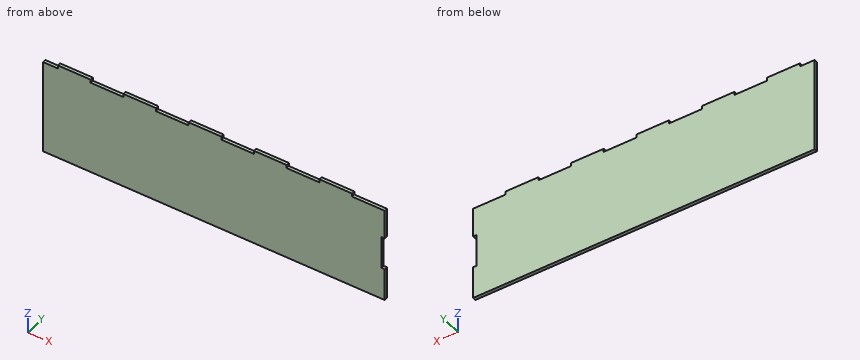
from build123d import *

# Parameters (mm, degrees)
SKETCH1_W              = 630
SKETCH1_H              = 90
BOSS_EXTRUDE1_DEPTH    = 3
SKETCH3_W              = 30
SKETCH3_H              = 3
CUT_EXTRUDE1_DEPTH     = 3
LPATTERN1_COUNT        = 10
LPATTERN1_PITCH        = 60
LPATTERN1_COL_COUNT    = 2
LPATTERN1_COL_PITCH    = 60
CUT_EXTRUDE5_START     = -3
CUT_EXTRUDE5_OUTLINE_W = 3
CUT_EXTRUDE5_OUTLINE_H = 30
CUT_EXTRUDE5_DEPTH     = 3
SKETCH7_W              = 3
SKETCH7_H              = 30
CUT_EXTRUDE3_DEPTH     = 3
SKETCH13_W             = 3
SKETCH13_H             = 27
CUT_EXTRUDE4_DEPTH     = 10


# Read off the part's stored shape, not the designer's step: Cut-Extrude5
with BuildPart() as part:
    # Sketch1 → Boss-Extrude1 (new body)
    with BuildSketch(Plane(origin=(0, 0, 0), x_dir=(1, 0, 0), z_dir=(0, 1, 0))):
        Rectangle(SKETCH1_W, SKETCH1_H)
    extrude(amount=BOSS_EXTRUDE1_DEPTH)

    # Sketch3 → Cut-Extrude1 (cut)
    with BuildSketch(Plane(origin=(0, 3, 0), x_dir=(1, 0, 0), z_dir=(0, 1, 0))):
        with Locations((-240, -43.5)):
            Rectangle(SKETCH3_W, SKETCH3_H)
    cut_extrude1 = extrude(amount=-CUT_EXTRUDE1_DEPTH, mode=Mode.SUBTRACT)

    # LPattern1: Cut-Extrude1 ×10
    with Locations(*[(i * LPATTERN1_PITCH, 0, 0) for i in range(1, LPATTERN1_COUNT)]):
        add(cut_extrude1, mode=Mode.SUBTRACT)

    # LPattern1 col: Cut-Extrude1 ×2
    with Locations(*[(-i * LPATTERN1_COL_PITCH, 0, 0) for i in range(1, LPATTERN1_COL_COUNT)]):
        add(cut_extrude1, mode=Mode.SUBTRACT)

    # Cut-Extrude5 outline → Cut-Extrude5 (cut)
    with BuildSketch(Plane(origin=(0, 3, 0), x_dir=(1, 0, 0), z_dir=(0, 1, 0)).offset(CUT_EXTRUDE5_START)):
        with Locations((313.5, 1e-09)):
            Rectangle(CUT_EXTRUDE5_OUTLINE_W, CUT_EXTRUDE5_OUTLINE_H)
    extrude(amount=CUT_EXTRUDE5_DEPTH, mode=Mode.SUBTRACT)

    # Sketch7 → Cut-Extrude3 (cut)
    with BuildSketch(Plane(origin=(0, 3, 0), x_dir=(1, 0, 0), z_dir=(0, 1, 0))):
        with Locations((-313.5, 30)):
            Rectangle(SKETCH7_W, SKETCH7_H)
    extrude(amount=-CUT_EXTRUDE3_DEPTH, mode=Mode.SUBTRACT)

    # Sketch13 → Cut-Extrude4 (cut)
    with BuildSketch(Plane(origin=(0, 3, 0), x_dir=(1, 0, 0), z_dir=(0, 1, 0))):
        with Locations((-313.5, -28.5)):
            Rectangle(SKETCH13_W, SKETCH13_H)
    extrude(amount=-CUT_EXTRUDE4_DEPTH, mode=Mode.SUBTRACT)

    # SurfaceCut1
    split(bisect_by=Plane.ZY.offset(-1.295), keep=Keep.BOTTOM)


solid = part.part
Here's how the part is built. I have some questions about the finished solid (model axes, mm). Give positions to 0.01 mm unless a question says otherwise; leave off trailing zeros. Loops run counter-clockwise (first coordinate to the right, second up) from the corner with the lowest first, then second, coordinate; pieces in that order, holes last. Notation, with made-up numbers: (86, 41.25) -> (95, 41.25) arc R23 ccw to (95, 59.25) -> close; hole circle Ø5 at (-21, 71). An arc over 180 degrees is marked (long way). One line per item, written item: value.
Q1. I'm going to push flat-ended pins straight in: pin 1 Ø1.5 at (y, z) = (1, 43.5) entering from +X; pin 2 Ø1.5 at (y, z) = (2, 44) entering from -X; pin 3 Ø1.5 at (x, y) = (300, 1.5) entering from +Z. Where does each tip first touch, or does it pass through?
Answers follow:
pin 1: x = 285
pin 2: x = 15
pin 3: z = 42
Q2. If I drill on line 1 along Z through (x, y) = (113.5, 0.8); line 2 along X through (y, z) = (2, -1) (3 decimals), over which ranges is the centre line in solid material (lowest first)?
Answers follow:
line 1: -45 to 42
line 2: 1.295 to 312
Q3. Suppose I cut it at B-B on x = 129. Please give me the cut outline in (y, z).
Answers follow:
outline: (0, -45) -> (3, -45) -> (3, 42) -> (0, 42) -> close
Q4. Suppose I cut it at A-A on y = 1. Please give me the cut outline in (x, z) (3 decimals), then the cut area to 3 significant figures.
Answers follow:
outline: (1.295, -45) -> (315, -45) -> (315, -15) -> (312, -15) -> (312, 15) -> (315, 15) -> (315, 42) -> (285, 42) -> (285, 45) -> (255, 45) -> (255, 42) -> (225, 42) -> (225, 45) -> (195, 45) -> (195, 42) -> (165, 42) -> (165, 45) -> (135, 45) -> (135, 42) -> (105, 42) -> (105, 45) -> (75, 45) -> (75, 42) -> (45, 42) -> (45, 45) -> (15, 45) -> (15, 42) -> (1.295, 42) -> close
area: 27,700 mm^2
